Drawing for the job (mm, zero at the part's lowest x, y, z). A direction names the side the tool comes from. Round coordinates to 2 decimals unless told otherwise and drop trailing zeros. Write each loop counter-clockwise with the first axis right and the second up, starting at its lowest first coordinate (ties: lowest second). Pieces come first, ordered by that corner, then holes. Notation, with made-up numbers: (-23, -15.75) -> (-10, -15.75) arc R18 cw to (-10, 14.25) -> close; hole circle Ø6 at (-27.75, 71.25). An arc over 180 degrees is marked (long way). Answer in a Markdown table with one row per item. Add a question column.
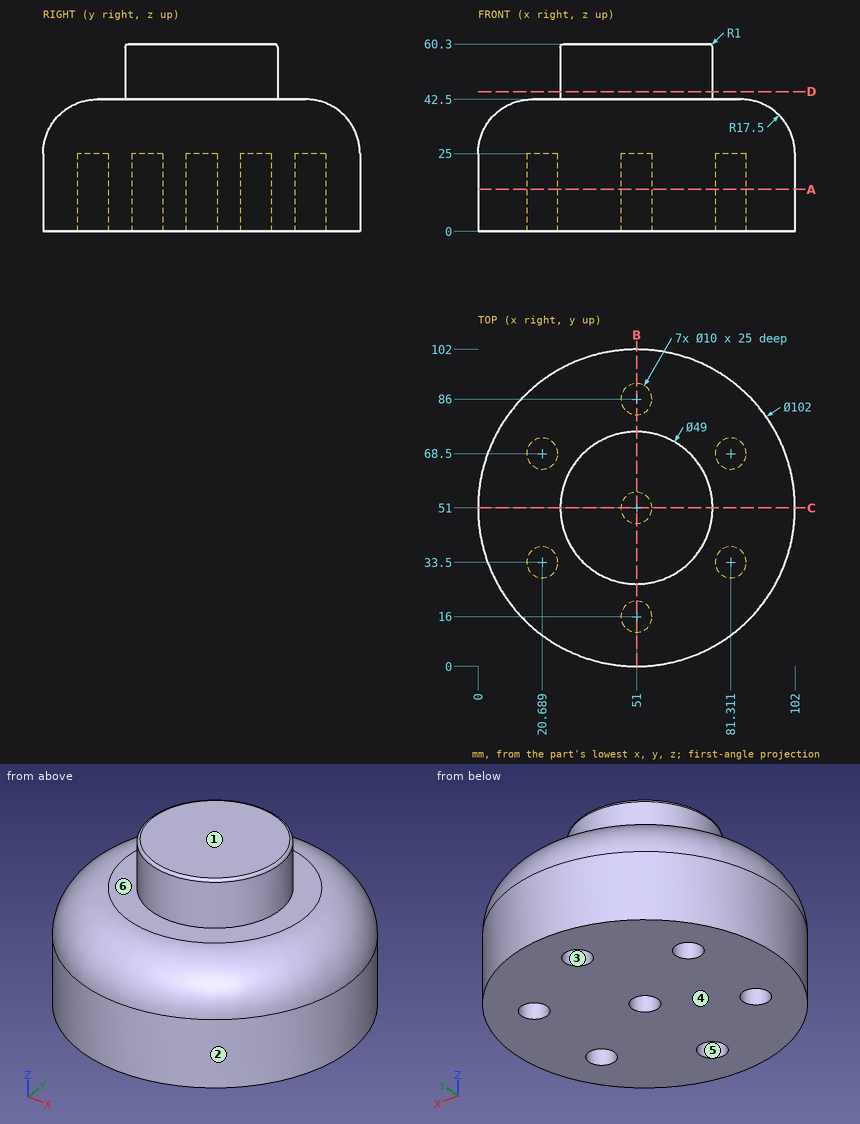
(1) Which spindle directions (+Z, -Z, +X, -X, +Y, -Y) get a long thin tool onto all of the face, cutting with end or side? Do the marked faces 4, 5 and 6. Say none if no direction does.
(2) Mould opens along X. For the marked faces 1, 2 and 3 say: pulls with the +X half, pulls with the -X half, needs draft (parallel to the pull), parting line crosses it, or undercut.
(3) Saw through at B-B (x = 51). List the corners of the cut face in (y, z), plus the area to 3 significant figures.
(4) Drop flat-ended pins along their axis: P1, Ø2, axis at y = 20, z = 30.5, coming from the -X side; P2, Ø6, axis at x = 20.69, y = 68.5, coming from the -Z side; P3, Ø13, axis at x = 51, y = 16, coming from the +Z side. Give the stop position or say it passes through.
(5) Saw through at A-A (z = 13.5). List the corners of the cut face in (x, y).
(6) Probe line 1 along Y through (x, z) = (51, 8); line 2 along X through (y, z) = (36, 22.5); line 3 along Y through (x, z) = (82, 14). List the from-to ranges inside material, lowest first.
(7) Saw through at D-D (z = 45). List the corners of the cut face in (x, y), plus the area to 3 significant figures.
(8) Saw through at C-C (y = 51). List the corners of the cut face in (x, z).
Answer sheet:
| question | item | result |
|---|---|---|
| 1 | face 4 | -Z, +X, -X, +Y, -Y |
| 1 | face 5 | -Z |
| 1 | face 6 | +Z |
| 2 | face 1 | needs draft |
| 2 | face 2 | parting line crosses it |
| 2 | face 3 | undercut |
| 3 | outline | (0, 0) -> (11, 0) -> (11, 25) -> (21, 25) -> (21, 0) -> (46, 0) -> (46, 25) -> (56, 25) -> (56, 0) -> (81, 0) -> (81, 25) -> (91, 25) -> (91, 0) -> (102, 0) -> (102, 25) arc R17.5 ccw to (84.5, 42.5) -> (75.5, 42.5) -> (75.5, 59.3) arc R1 ccw to (74.5, 60.3) -> (27.5, 60.3) arc R1 ccw to (26.5, 59.3) -> (26.5, 42.5) -> (17.5, 42.5) arc R17.5 ccw to (0, 25) -> close |
| 3 | area | 4,330 mm² |
| 4 | P1 | stops at x = 10.76 |
| 4 | P2 | stops at z = 25 |
| 4 | P3 | stops at z = 42.5 |
| 5 | outline | circle Ø102 at (51, 51); hole circle Ø10 at (20.69, 33.5); hole circle Ø10 at (20.69, 68.5); hole circle Ø10 at (51, 16); hole circle Ø10 at (51, 51); hole circle Ø10 at (51, 86); hole circle Ø10 at (81.31, 33.5); hole circle Ø10 at (81.31, 68.5) |
| 6 | line 1 | y = 0 to 11, 21 to 46, 56 to 81, 91 to 102 |
| 6 | line 2 | x = 2.26 to 16.36, 25.02 to 76.98, 85.64 to 99.74 |
| 6 | line 3 | y = 10.5 to 28.55, 38.45 to 63.55, 73.45 to 91.5 |
| 7 | outline | circle Ø49 at (51, 51) |
| 7 | area | 1,890 mm² |
| 8 | outline | (0, 0) -> (46, 0) -> (46, 25) -> (56, 25) -> (56, 0) -> (102, 0) -> (102, 25) arc R17.5 ccw to (84.5, 42.5) -> (75.5, 42.5) -> (75.5, 59.3) arc R1 ccw to (74.5, 60.3) -> (27.5, 60.3) arc R1 ccw to (26.5, 59.3) -> (26.5, 42.5) -> (17.5, 42.5) arc R17.5 ccw to (0, 25) -> close |
